```python
from build123d import *

# Parameters (mm, degrees)
Y_KSEKLIK_EKSTR_ZYON2_DEPTH = 77
IZIM3_W                     = 2
IZIM3_H                     = 1.25
KES_EKSTR_ZYON1_DEPTH       = 77
IZIM6_W                     = 1.5
IZIM6_H                     = 74.5
Y_KSEKLIK_EKSTR_ZYON3_DEPTH = 2
IZIM7_W                     = 7
IZIM7_H                     = 10
KES_EKSTR_ZYON2_DEPTH       = 10


with BuildPart() as part:
    # Çizim2 → Yükseklik-Ekstrüzyon2 (new body)
    with BuildSketch(Plane.XY):
        Polygon((55.5, 40), (-55.5, 40), (-55.5, -40), (55.5, -40), (55.5, -36), (-51.5, -36), (-51.5, 36), (55.5, 36), align=None)
    extrude(amount=-Y_KSEKLIK_EKSTR_ZYON2_DEPTH)

    # Çizim3 → Kes-Ekstrüzyon1 (cut)
    with BuildSketch(Plane(origin=(0, 0, -77), x_dir=(-1, 0, 0), z_dir=(0, 0, -1))):
        with Locations((-54.5, -36.625)):
            Rectangle(IZIM3_W, IZIM3_H)
        with Locations((-54.5, -39.375)):
            Rectangle(IZIM3_W, IZIM3_H)
        with Locations((-54.5, 39.375)):
            Rectangle(IZIM3_W, IZIM3_H)
        with Locations((-54.5, 36.625)):
            Rectangle(IZIM3_W, IZIM3_H)
    extrude(amount=-KES_EKSTR_ZYON1_DEPTH, mode=Mode.SUBTRACT)

    # Çizim6 → Yükseklik-Ekstrüzyon3 (add)
    with BuildSketch(Plane(origin=(0, 0, -77), x_dir=(-1, 0, 0), z_dir=(0, 0, -1))):
        Polygon((-53.5, 38.75), (-55.5, 38.75), (-55.5, 37.25), (-53.5, 37.25), (52.75, 37.25), (54.25, 37.25), (54.25, 38.75), align=None)
        with Locations((53.5, 0)):
            Rectangle(IZIM6_W, IZIM6_H)
        Polygon((54.25, -38.75), (54.25, -37.25), (52.75, -37.25), (-53.5, -37.25), (-55.5, -37.25), (-55.5, -38.75), (-53.5, -38.75), align=None)
    extrude(amount=Y_KSEKLIK_EKSTR_ZYON3_DEPTH)

    # Çizim7 → Kes-Ekstrüzyon2 (cut)
    with BuildSketch(Plane.XZ.offset(40)):
        with Locations((-46, -74)):
            Rectangle(IZIM7_W, IZIM7_H)
    extrude(amount=-KES_EKSTR_ZYON2_DEPTH, mode=Mode.SUBTRACT)


solid = part.part
```
Can you work these out from the model? Positions are in its coordinate system, mm. A direction names the side the tool comes from. Round coordinates to 2 decimals unless told otherwise and drop trailing zeros. Loops run counter-clockwise (first coordinate to the right, second up) from the corner with the lowest first, then second, coordinate; pieces in that order, holes last.
Item 1: Suppose I cut it at C-C, the plane y = -7. Write out the boundary of the cut face in (x, z), then the cut area to 3 significant figures.
Item 2: If we mould it in two halves opening along X, with no side actions, what happens to faces 6 (the flat face through (-46, -38, -69)), 7 (the flat face through (0, 36, -38)), 8 (the flat face through (-51.5, -1, -38)), 9 (the flat face through (-49.5, -38, -73))? For each: +X half, -X half, draft (parallel to the pull), parting line (faces both ways), or undercut.
Item 3: Will these pins go through, and if not, where does the flat tip stop? pin 1 Ø0.6 at (x, z) = (-50.5, -78.5) entering from +Y; pin 2 Ø1 at (y, z) = (0, -78) entering from -X; pin 3 Ø10 at (y, z) = (1, -30) entering from +X.
Item 4: Suppose I cut it at A-A, the plane x = -3.5. Write out the boundary of the cut face in (y, z), then the cut area to 3 significant figures.
Item 5: Suppose I cut it at B-B, the plane z = -38.5. Write out the boundary of the cut face in (x, y).
Item 6: Which directions (+Z, -Z, +X, -X, +Y, -Y) give clear straight access to the entire face, cutting with the end or side of a thin tool? Please do faces 1 (the flat face through (-2, -40, -38)), 2 (the flat face through (-55.5, 1, -38)), 3 (the flat face through (25.7, 37.25, -77.4)), 4 (the flat face through (-42.5, -38, -73)), 5 (the flat face through (2, -36, -38)).
Item 7: Please list where these lines run through material, in increasing order: L1, parallel to Y at x = -5, z = -7; L2, parallel to X at y = 13.5, z = -27.5; L3, parallel to X at y = 37, z = -12.
Reported:
1. outline: (-55.5, -77) - (-54.25, -77) - (-54.25, -79) - (-52.75, -79) - (-52.75, -77) - (-51.5, -77) - (-51.5, 0) - (-55.5, 0) - close
1. area: 311 mm2
2. face 6: undercut
2. face 7: draft
2. face 8: +X half
2. face 9: undercut
3. pin 1: stops at y = 38.75
3. pin 2: stops at x = -54.25
3. pin 3: stops at x = -51.5
4. outline: (-40, -77) - (-38.75, -77) - (-38.75, -79) - (-37.25, -79) - (-37.25, -77) - (-36, -77) - (-36, 0) - (-40, 0) - close; (36, -77) - (37.25, -77) - (37.25, -79) - (38.75, -79) - (38.75, -77) - (40, -77) - (40, 0) - (36, 0) - close
4. area: 622 mm2
5. outline: (-55.5, -40) - (53.5, -40) - (53.5, -38.75) - (55.5, -38.75) - (55.5, -37.25) - (53.5, -37.25) - (53.5, -36) - (-51.5, -36) - (-51.5, 36) - (53.5, 36) - (53.5, 37.25) - (55.5, 37.25) - (55.5, 38.75) - (53.5, 38.75) - (53.5, 40) - (-55.5, 40) - close
6. face 1: +Z, -Z, +X, -X, -Y
6. face 2: +Z, -Z, -X, +Y, -Y
6. face 3: -Z, +X
6. face 4: -Z, -Y
6. face 5: +Z, -Z, +X
7. L1: y = -40 to -36, 36 to 40
7. L2: x = -55.5 to -51.5
7. L3: x = -55.5 to 53.5
